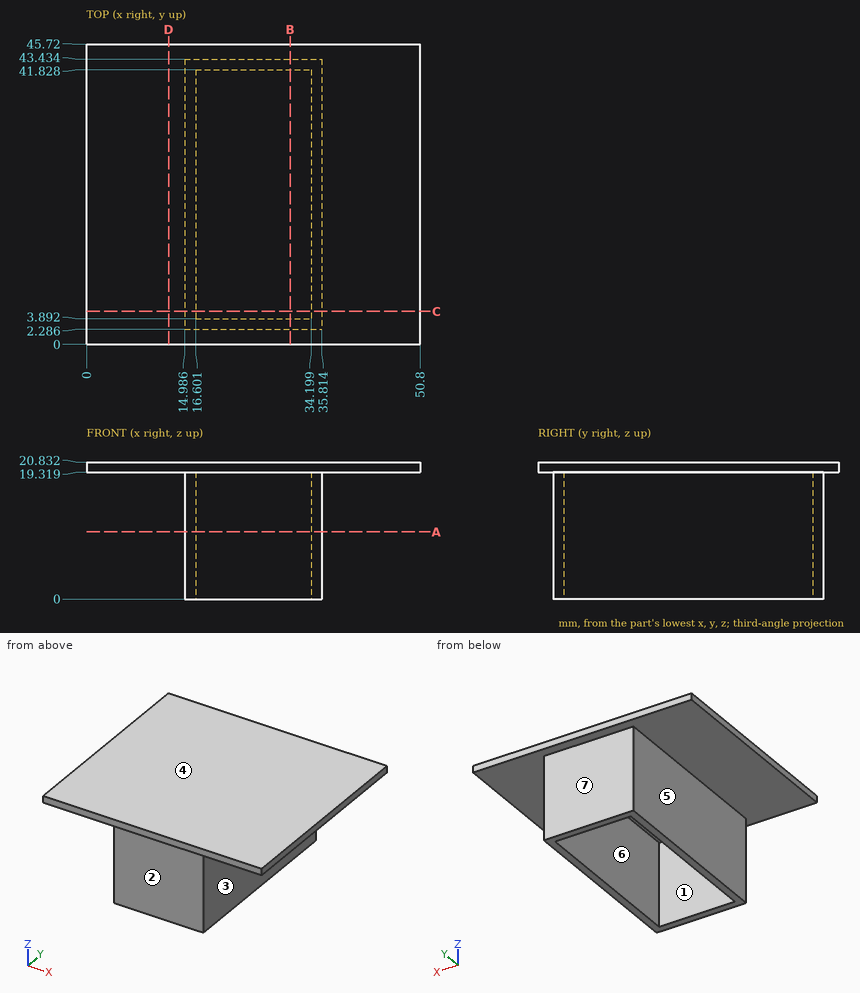
Part print with two shaded views. Sizes in mm from the minimum x, y, z corner. A direction names the side the tool comes from. Coordinates: 2 decimals unless noted, no trailing zeros. Loops run counter-clockwise (first coordinate to the right, second up) from the corner with the lowest first, then second, coordinate; pieces in that order, holes last. Notation, with made-up numbers: M 68,75.25 L 127,75.25 A23 cw 127,93.25 Z; hole C 44.5,79.5 d2. An arc over 180 degrees is marked long. Use CSV: the item, a comma, the result in double quotes. Start each with the question number.
1. Band-saw the part on C-C, the plane y = 5. List the corners of the cut face in (x, z), then the cut area to 3 significant figures.
2. Band-saw the part on B-B, the plane x = 31. List the corners of the cut face in (y, z).
3. Band-saw the part on A-A, the plane z = 10.25. List the corners of the cut face in (x, y).
4. Flat gauge pins, fed straight in: pin 1 (2 mm diameter, centred on x = 12, y = 37.5, fed in from -Z); pin 2 (9 mm diameter, centred on x = 21, z = 11.5, fed in from -Y); pin 3 (1 mm diameter, centred on x = 15, z = 10.5, fed in from +Y). Where does each tip first touch, or does it go through?
5. Two-plate mould, pull along X, no slides. Class the marked faces 1, 2 and 3: pulls with the +X half, pulls with the -X half, needs draft (parallel to the pull), parting line crosses it, or undercut.
6. Band-saw the part on D-D, the plane x = 12.5. List the corners of the cut face in (y, z).
7. Probe probe 1 along X at (y, z) = (19.5, 1.5); probe 2 along Y at (x, z) = (30, 6.5); probe 3 along Z at (x, y) = (13.5, 19.5). List the from-to ranges inside material, lowest first. Write a range as [from, to].
8. Tool access for the marked faces 4, 5, 6 and 7: list every direction of +Z, -Z, +X, -X, +Y, -Y with a clear straight run to the whole face (end or side of a thin tool).
Entries:
1,outline,"M 0,19.32 L 14.99,19.32 L 14.99,0 L 16.6,0 L 16.6,19.32 L 34.2,19.32 L 34.2,0 L 35.81,0 L 35.81,19.32 L 50.8,19.32 L 50.8,20.83 L 0,20.83 Z"
1,area,"139 mm2"
2,outline,"M 0,19.32 L 2.29,19.32 L 2.29,0 L 3.89,0 L 3.89,19.32 L 41.83,19.32 L 41.83,0 L 43.43,0 L 43.43,19.32 L 45.72,19.32 L 45.72,20.83 L 0,20.83 Z"
3,outline,"M 14.99,2.29 L 35.81,2.29 L 35.81,43.43 L 14.99,43.43 Z; hole M 16.6,3.89 L 34.2,3.89 L 34.2,41.83 L 16.6,41.83 Z"
4,pin 1,"stops at z = 19.32"
4,pin 2,"stops at y = 2.29"
4,pin 3,"stops at y = 43.43"
5,face 1,"undercut"
5,face 2,"needs draft"
5,face 3,"pulls with the +X half"
6,outline,"M 0,19.32 L 45.72,19.32 L 45.72,20.83 L 0,20.83 Z"
7,probe 1,"x = [14.99, 16.6], [34.2, 35.81]"
7,probe 2,"y = [2.29, 3.89], [41.83, 43.43]"
7,probe 3,"z = [19.32, 20.83]"
8,face 4,"+Z, +X, -X, +Y, -Y"
8,face 5,"-Z, -X, +Y, -Y"
8,face 6,"-Z"
8,face 7,"-Z, +X, -X, +Y"
